```python
from build123d import *

# Parameters (mm, degrees)
ESQUISSE1_R             = 5.5
ESQUISSE1_W             = 6
ESQUISSE1_H             = 6
BASE_EXTRUSION_DEPTH    = 4
ESQUISSE2_W             = 6
ESQUISSE2_H             = 6
BOSS_EXTRU_1_DEPTH      = 1.5
ESQUISSE3_R             = 1.5
ENL_V_MAT_EXTRU_1_DEPTH = 6.5
ESQUISSE6_R             = 2.5
CONG_1_R                = 2.5
ESQUISSE7_R             = 0.75
ENL_V_MAT_EXTRU_2_DEPTH = 11.5
BOSS_EXTRU_2_DEPTH      = 1


with BuildPart() as part:
    # Esquisse1 → Base-Extrusion (new body, symmetric)
    with BuildSketch(Plane.XY):
        Circle(ESQUISSE1_R)
        Rectangle(ESQUISSE1_W, ESQUISSE1_H, mode=Mode.SUBTRACT)
    extrude(amount=BASE_EXTRUSION_DEPTH, both=True)

    # Esquisse2 → Boss.-Extru.1 (add, symmetric)
    with BuildSketch(Plane.XY):
        Rectangle(ESQUISSE2_W, ESQUISSE2_H)
    extrude(amount=BOSS_EXTRU_1_DEPTH, both=True)

    # Esquisse3 → Enl_v. mat.-Extru.1 (cut, through all)
    with BuildSketch(Plane.XY.offset(1.5)):
        Circle(ESQUISSE3_R)
    extrude(amount=-ENL_V_MAT_EXTRU_1_DEPTH, mode=Mode.SUBTRACT)

    # Boss.-Balayage1: sweep along a curve in space
    with BuildLine() as boss_balayage1_path:
        Line((-3.728314003, 0.998998726, 0), (-26.294095226, 7.045481581, 0))
        ThreePointArc((-26.294095226, 7.045481581, 0), (-28.966766701, 8.831303568, 0), (-30, 11.875110713, 0))
        Line((-30, 11.875110713, 0), (-30, 70, 0))
    # Esquisse6 → Boss.-Balayage1 (sweep)
    with BuildSketch(Plane(origin=(0, 70, 0), x_dir=(-1, 0, 0), z_dir=(0, 1, 0))):
        with Locations((30, 0)):
            Circle(ESQUISSE6_R)
    sweep(path=boss_balayage1_path.line)

    # Cong_1
    cong_1_edges = [part.edges().sort_by_distance(p)[0] for p in [
        (-27.5, 70, 0),
    ]]
    fillet(cong_1_edges, radius=CONG_1_R)

    # Esquisse7 → Enl_v. mat.-Extru.2 (cut, symmetric)
    with BuildSketch(Plane.XY):
        with Locations((-30, 27)):
            Circle(ESQUISSE7_R)
        with Locations((-30, 32)):
            Circle(ESQUISSE7_R)
        with Locations((-30, 37)):
            Circle(ESQUISSE7_R)
        with Locations((-30, 42)):
            Circle(ESQUISSE7_R)
        with Locations((-30, 47)):
            Circle(ESQUISSE7_R)
        with Locations((-30, 52)):
            Circle(ESQUISSE7_R)
        with Locations((-30, 57)):
            Circle(ESQUISSE7_R)
        with Locations((-30, 62)):
            Circle(ESQUISSE7_R)
    extrude(amount=ENL_V_MAT_EXTRU_2_DEPTH, both=True, mode=Mode.SUBTRACT)

    # Esquisse8 → Boss.-Extru.2 (add, symmetric)
    with BuildSketch(Plane.XY):
        Polygon((0, 5.5), (-19, 7), (-2, 2), align=None)
    extrude(amount=BOSS_EXTRU_2_DEPTH, both=True)


solid = part.part
```
Input: part model. Units: mm. Frame: model coordinates. A direction names the side the tool comes from. Give positions to 0.01 mm unless a question says otherwise; leave off trailing zeros. Write each loop counter-clockwise with the first axis right and the second up, starting at its lowest first coordinate (ties: lowest second). Pieces come first, ordered by that corner, then holes. Notation, with made-up numbers: (14, 1.5) - (63, 1.5) arc R20 ccw to (63, 28.5) - close; hole circle Ø6 at (-15, -0.5). An arc over 180 degrees is marked (long way). Write item = value, one per line. Start each with the question number.
1) Cut plane B-B (y = 54). Return loops of the section in (x, z), and give its area (3 significant figures).
2) Draft query along X for faces 4 (the face through (-32.31, 40.08, -0.96)), 5 (the face through (-8, 5, -1)), 6 (the face through (-8, 5, 1)), 7 (the face through (4, 0, -4)). Return one class per face: pulls with the +X half, pulls with the -X half, needs draft (parallel to the pull), parting line crosses it, or undercut.
3) Cut plane A-A (x = -30). Give the number of separate pieces and of enclosed holes in the cut face, and give its area (3 significant figures).
4) Pin query (flat end, axial travel): pin 1 (5 mm diameter, centred on x = 1, y = 1, fed in from -Z); pin 2 (2 mm diameter, centred on x = -30, y = 52, fed in from -Z); pin 3 (2 mm diameter, centred on x = -30, y = 57, fed in from +Z); pin 4 (0.8 mm diameter, centred on x = -0.5, z = -2.5, fed in from +Y). Return the tip coordinate at first contact, or that it passes through.
5) Material intervals for L1, parallel to Z at x = -18.5, y = 5; L2, parallel to X at y = 21.5, z = -0.25; L3, parallel to X at y = 47, z = -1.75, sorted ascending. Write a range as [from, to].
6) Reachability of faces 1 (the face through (3, 0, 3)), 2 (the face through (-16.281, 1.894, 0.751)), 3 (the face through (-1.4, 1.4, -1.5)) from +Z, -Z, +X, -X, +Y, -Y: full face, straight path, thin tool, end or side. Return the list, or none.
Answers follow:
q1.outline = circle Ø5 at (-30, 0)
q1.area = 19.6 mm^2
q2.face_4 = parting line crosses it
q2.face_5 = undercut
q2.face_6 = undercut
q2.face_7 = needs draft
q3.separate_pieces = 9
q3.enclosed_holes = 0
q3.area = 252 mm^2
q4.pin_1 = -4
q4.pin_2 = -2.5
q4.pin_3 = 2.5
q4.pin_4 = 5.5
q5.L1 = [-2.5, 2.5]
q5.L2 = [-32.49, -27.51]
q5.L3 = [-31.79, -30.75], [-29.25, -28.21]
q6.face_1 = +Z
q6.face_2 = none
q6.face_3 = -Z
